Can you work these out from the model? Positions are in its coordinate system, mm. A direction names the side the tool comes from. Round coordinates to 2 decimals unless told otherwise and drop trailing zeros. Write each loop counter-clockwise with the first axis right and the second up, starting at its lowest first coordinate (ties: lowest second). Pieces come first, ordered by that corner, then holes.
Q1. For faces 5 (the flat face through (12.7, 32, 14)), 6 (the flat face through (3.81, 28, 3)), 7 (the flat face through (29, 6.35, 3)), which set-ups out of +Z, -Z, +X, -X, +Y, -Y let a thin tool reach every point of the face, with its end or its side?
Q2. We'd pull the mould along Z, two halves only. Please class faces 1 (the flat face through (50.8, 13, 9)), 2 (the flat face through (23, 23, 19.05)), 3 (the flat face through (23, 24, 0)), 4 (the flat face through (28, 23, 15.24)): +Z half, -Z half, draft (parallel to the pull), parting line (faces both ways), or undercut.
Q3. If we section it at B-B (y = 22.5): Please give me the cut outline in (x, z).
Q4. If we section it at D-D (z = 9.25): Please give me the cut outline in (x, y).
Q5. If we section it at C-C (x = 9.5): Please give me the cut outline in (y, z).
Q6. If we section it at A-A (z = 5.5): Please give me the cut outline in (x, y).
Q7. Please list where these lines run through material, in increasing order: line 1 along Z through (x, y) = (25, 45); line 2 along Y through (x, z) = (18, 6).
Q8. I'm going to push flat-ended pins straight in: pin 1 Ø4 at (y, z) = (43.5, 8) entering from +X; pin 2 Ø19 at (x, y) = (30.5, 34.5) entering from -Z; pin 3 Ø2 at (x, z) = (33.5, 14) entering from +Y; pin 4 Ø3 at (x, z) = (32, 18) entering from +Y. Where does each tip first touch, or does it pass through?
from build123d import *

# Parameters (mm, degrees)
F1_DEPTH = 19.05
F2_W     = 2.54
F2_H     = 6.35
F3_DEPTH = 46.99
F2_W_2   = 12.7
F2_H_2   = 2.54
F4_DEPTH = 38.1
F5_W     = 12.7
F5_H     = 2.54
F6_DEPTH = 38.1
F5_W_2   = 2.54
F5_H_2   = 6.35
F7_DEPTH = 46.736
F8_R     = 5.08


with BuildPart() as f1:
    # F0 (on Top) → F1 (new body)
    with BuildSketch(Plane.XY):
        Polygon((0, 25.4), (0, 0), (25.4, 0), (50.8, 0), (50.8, 25.4), (25.4, 25.4), (25.4, 50.8), (0, 50.8), align=None)
    extrude(amount=F1_DEPTH)

    # F2 (on face) → F3 (cut)
    with BuildSketch(Plane.YZ.offset(50.8)):
        with Locations((5.08, 3.175)):
            Rectangle(F2_W, F2_H)
    extrude(amount=-F3_DEPTH, mode=Mode.SUBTRACT)

    # F2 (on face) → F4 (cut)
    with BuildSketch(Plane.YZ.offset(50.8)):
        with Locations((19.05, 13.97)):
            Rectangle(F2_W_2, F2_H_2)
    extrude(amount=-F4_DEPTH, mode=Mode.SUBTRACT)

    # F5 (on face) → F6 (cut)
    with BuildSketch(Plane(origin=(0, 50.8, 0), x_dir=(-1, 0, 0), z_dir=(0, 1, 0))):
        with Locations((-19.05, 13.97)):
            Rectangle(F5_W, F5_H)
    extrude(amount=-F6_DEPTH, mode=Mode.SUBTRACT)

    # F5 (on face) → F7 (cut)
    with BuildSketch(Plane(origin=(0, 50.8, 0), x_dir=(-1, 0, 0), z_dir=(0, 1, 0))):
        with Locations((-5.08, 3.175)):
            Rectangle(F5_W_2, F5_H_2)
    extrude(amount=-F7_DEPTH, mode=Mode.SUBTRACT)

    # F8
    f8_edges = [f1.edges().sort_by_distance(p)[0] for p in [
        (25.4, 0, 19.05),
        (0, 25.4, 19.05),
    ]]
    fillet(f8_edges, radius=F8_R)


solid = f1.part
A:
1. face 5: +X, +Y
1. face 6: -Z, +Y
1. face 7: -Z, +X
2. face 1: draft
2. face 2: +Z half
2. face 3: -Z half
2. face 4: undercut
3. outline: (0, 0) - (3.81, 0) - (3.81, 6.35) - (6.35, 6.35) - (6.35, 0) - (50.8, 0) - (50.8, 12.7) - (12.7, 12.7) - (12.7, 15.24) - (50.8, 15.24) - (50.8, 19.05) - (5.08, 19.05) arc R5.08 ccw to (0, 13.97) - close
4. outline: (0, 0) - (50.8, 0) - (50.8, 25.4) - (25.4, 25.4) - (25.4, 50.8) - (0, 50.8) - close
5. outline: (0, 0) - (3.81, 0) - (3.81, 6.35) - (6.35, 6.35) - (6.35, 0) - (50.8, 0) - (50.8, 19.05) - (5.08, 19.05) arc R5.08 ccw to (0, 13.97) - close
6. outline: (0, 0) - (50.8, 0) - (50.8, 3.81) - (3.81, 3.81) - (3.81, 50.8) - (0, 50.8) - close; (6.35, 6.35) - (50.8, 6.35) - (50.8, 25.4) - (25.4, 25.4) - (25.4, 50.8) - (6.35, 50.8) - close
7. line 1: z = 0 to 12.7, 15.24 to 19.05
7. line 2: y = 0 to 3.81, 6.35 to 50.8
8. pin 1: stops at x = 25.4
8. pin 2: stops at z = 0
8. pin 3: stops at y = 12.7
8. pin 4: stops at y = 25.4
